from build123d import *

# Parameters (mm, degrees)
EXTRUDE_1_DEPTH          = 419
CUT_EXTRUDE_START        = -20
SKETCH_2_R               = 119
SKETCH_2_R_2             = 99
CUT_EXTRUDE_1_DEPTH      = 379
SKETCH_3_R               = 93
CUT_EXTRUDE_2_DEPTH      = 420
SKETCH_4_W               = 17.5
SKETCH_4_H               = 1
SKETCH_4_W_2             = 1
SKETCH_4_H_2             = 15.5
SKETCH_4_W_3             = 15.5
CUT_EXTRUDE_3_DEPTH      = 420
SKETCH_5_R               = 3
CUT_EXTRUDE_4_DEPTH      = 12.158706001
PATTERN_CIRCULAR_1_COUNT = 4


with BuildPart() as part:
    # 草图1 → 凸台-拉伸1 (new body)
    with BuildSketch(Plane.XY):
        with BuildLine():
            Line((-9.75, -98.518716496), (-9.75, -105.83522676))
            Line((-9.75, -105.83522676), (9.75, -105.83522676))
            Line((9.75, -105.83522676), (9.75, -98.518716496))
            ThreePointArc((9.75, -98.518716496), (70.003571337, -70.003571337), (98.518716496, -9.75))
            Line((98.518716496, -9.75), (104.83522676, -9.75))
            Line((104.83522676, -9.75), (104.83522676, 9.75))
            Line((104.83522676, 9.75), (98.518716496, 9.75))
            ThreePointArc((98.518716496, 9.75), (70.003571337, 70.003571337), (9.75, 98.518716496))
            Line((9.75, 98.518716496), (9.75, 104.83522676))
            Line((9.75, 104.83522676), (-9.75, 104.83522676))
            Line((-9.75, 104.83522676), (-9.75, 98.518716496))
            ThreePointArc((-9.75, 98.518716496), (-70.003571337, 70.003571337), (-98.518716496, 9.75))
            Line((-98.518716496, 9.75), (-104.83522676, 9.75))
            Line((-104.83522676, 9.75), (-104.83522676, -9.75))
            Line((-104.83522676, -9.75), (-98.518716496, -9.75))
            ThreePointArc((-98.518716496, -9.75), (-70.003571337, -70.003571337), (-9.75, -98.518716496))
        make_face()
    extrude(amount=EXTRUDE_1_DEPTH)

    # 草图2 → 切除-拉伸1 (cut)
    with BuildSketch(Plane.XY.offset(419).offset(CUT_EXTRUDE_START)):
        Circle(SKETCH_2_R)
        Circle(SKETCH_2_R_2, mode=Mode.SUBTRACT)
    extrude(amount=-CUT_EXTRUDE_1_DEPTH, mode=Mode.SUBTRACT)

    # 草图3 → 切除-拉伸2 (cut, through all)
    with BuildSketch(Plane.XY.offset(419)):
        Circle(SKETCH_3_R)
    extrude(amount=-CUT_EXTRUDE_2_DEPTH, mode=Mode.SUBTRACT)

    # 草图4 → 切除-拉伸3 (cut, through all)
    with BuildSketch(Plane.XY.offset(419)):
        with Locations((0, -93.087458654)):
            Rectangle(SKETCH_4_W, SKETCH_4_H)
        with Locations((-93.176520759, 0)):
            Rectangle(SKETCH_4_W_2, SKETCH_4_H_2)
        with Locations((0, 93.176520759)):
            Rectangle(SKETCH_4_W_3, SKETCH_4_H)
        with Locations((93.176520759, 0)):
            Rectangle(SKETCH_4_W_2, SKETCH_4_H_2)
    extrude(amount=-CUT_EXTRUDE_3_DEPTH, mode=Mode.SUBTRACT)

    # 草图5 → 切除-拉伸4 (cut, through all)
    with BuildSketch(Plane(origin=(-93.676520759, 0, 0), x_dir=(0, 0, -1), z_dir=(1, 0, 0))):
        with Locations((-409, 0)):
            Circle(SKETCH_5_R)
        with Locations((-10, 0)):
            Circle(SKETCH_5_R)
    cut_extrude_4 = extrude(amount=-CUT_EXTRUDE_4_DEPTH, mode=Mode.SUBTRACT)

    # 阵列(圆周)1: 切除-拉伸4 ×4 about axis
    pattern_circular_1_axis = Axis((0, 0, 1000), (0, 0, -1))
    for i in range(1, PATTERN_CIRCULAR_1_COUNT):
        add(cut_extrude_4.rotate(pattern_circular_1_axis, i * 360 / PATTERN_CIRCULAR_1_COUNT), mode=Mode.SUBTRACT)


solid = part.part
Work out the finished part from the listing and answer in its coordinate system (mm). A direction names the side the tool comes from. Coordinates: 2 decimals unless noted, no trailing zeros. Loops run counter-clockwise (first coordinate to the right, second up) from the corner with the lowest first, then second, coordinate; pieces in that order, holes last. Notation, with made-up numbers: (84, -36.75) -> (118, -36.75) arc R33 ccw to (118, -1.75) -> close; hole circle Ø4 at (-26.5, 4.25). An arc over 180 degrees is marked (long way). Write each question's results on one line, items separated by ' | '. Start each with the question number.
1) The mould has two halves that part along X. Classify faces 1 (the cylindrical face through (66.404, 65.111, 212.433)), 2 (the flat face through (-104.835, 2.3, 406.6)), 3 (the flat face through (62, -70, 419)): pulls with the +X half, pulls with the -X half, needs draft (parallel to the pull), parting line crosses it, or undercut.
2) Find section B-B on y = 26.5. Determine the outline of the cut face in (x, z), then the cut area to 3 significant figures.
3) For faces 4 (the flat face through (0, -93.587, 212)), 5 (the flat face through (2.3, 104.835, 406.6)), determine the directions among +Z, -Z, +X, -X, +Y, -Y from which every point of the face is accessible in a straight line to the end or side of a thin tool.
4) Find section A-A on z = 250.5. Determine the outline of the cut face in (x, y).
5) Consider line 1 along Z through (x, y) = (0, 100); line 2 along Y through (x, z) = (102.25, 10). Determine where each line is inside the solid, lowest interval first.
6) Find section C-C on x = 62. Determine the outline of the cut face in (y, z), then the cut area to 3 significant figures.
7) Flat-ended cylindrical pins translate along their axes: P1, Ø5, axis at y = -4.5, z = 238.5, coming from the +X side; P2, Ø5, axis at y = 27.5, z = 264, coming from the +X side; P3, Ø10, axis at y = 33.5, z = 92.5, coming from the -X side. Find the tip coordinate at first contact, or state that the pin passes through.
Response values:
1) face 1: undercut | face 2: pulls with the -X half | face 3: needs draft
2) outline: (-95.39, 0) -> (-89.14, 0) -> (-89.14, 419) -> (-95.39, 419) -> close; (89.14, 0) -> (95.39, 0) -> (95.39, 419) -> (89.14, 419) -> close | area: 5,230 mm^2
3) face 4: +Z, -Z | face 5: +Z, -Z, +X, -X, +Y
4) outline: circle Ø198 at (0, 0); hole (-93.68, -7.75) -> (-92.68, -7.75) arc R93 ccw to (-8.75, -92.59) -> (-8.75, -93.59) -> (8.75, -93.59) -> (8.75, -92.59) arc R93 ccw to (92.68, -7.75) -> (93.68, -7.75) -> (93.68, 7.75) -> (92.68, 7.75) arc R93 ccw to (7.75, 92.68) -> (7.75, 93.68) -> (-7.75, 93.68) -> (-7.75, 92.68) arc R93 ccw to (-92.68, 7.75) -> (-93.68, 7.75) -> close
5) line 1: z = 0 to 7, 13 to 20, 399 to 406, 412 to 419 | line 2: y = -9.75 to -3, 3 to 9.75
6) outline: (-77.18, 0) -> (-69.32, 0) -> (-69.32, 419) -> (-77.18, 419) -> close; (69.32, 0) -> (77.18, 0) -> (77.18, 419) -> (69.32, 419) -> close | area: 6,590 mm^2
7) P1: stops at x = 98.98 | P2: stops at x = 95.79 | P3: stops at x = -94.81
